from build123d import *

# Parameters (mm, degrees)
SKETCH1_W           = 12.1
SKETCH1_H           = 11.4
BOSS_EXTRUDE1_DEPTH = 500
SKETCH2_R           = 3.379
SKETCH2_R_2         = 1.9
CUT_EXTRUDE1_DEPTH  = 501.069087727
FILLET1_R           = 0.2


with BuildPart() as part:
    # Sketch1 → Boss-Extrude1 (new body)
    with BuildSketch(Plane.XY):
        Rectangle(SKETCH1_W, SKETCH1_H)
    extrude(amount=BOSS_EXTRUDE1_DEPTH)

    # Sketch2 → Cut-Extrude1 (cut, through all)
    with BuildSketch(Plane.XY.offset(500)):
        with Locations((0, 7.279)):
            Circle(SKETCH2_R)
        with Locations((0, -7.279)):
            Circle(SKETCH2_R)
        with Locations((-6.565, 2.930166572)):
            Circle(SKETCH2_R_2)
        with Locations((-6.565, -2.930166572)):
            Circle(SKETCH2_R_2)
        with Locations((6.565, -2.930166572)):
            Circle(SKETCH2_R_2)
        with Locations((6.565, 2.930166572)):
            Circle(SKETCH2_R_2)
    extrude(amount=-CUT_EXTRUDE1_DEPTH, mode=Mode.SUBTRACT)

    # Fillet1
    fillet1_edges = [part.edges().sort_by_distance(p)[0] for p in [
        (6.05, -4.759039176, 250),
        (6.05, -1.101293968, 250),
        (-6.05, -1.101293968, 250),
        (-6.05, -4.759039176, 250),
        (-6.05, 4.759039176, 250),
        (-6.05, 1.101293968, 250),
        (-2.987373428, -5.7, 250),
        (2.987373428, -5.7, 250),
        (6.05, 1.101293968, 250),
        (6.05, 4.759039176, 250),
        (2.987373428, 5.7, 250),
        (-2.987373428, 5.7, 250),
        (6.05, -5.7, 250),
        (-6.05, -5.7, 250),
        (-6.05, 5.7, 250),
        (6.05, 5.7, 250),
    ]]
    fillet(fillet1_edges, radius=FILLET1_R)


solid = part.part
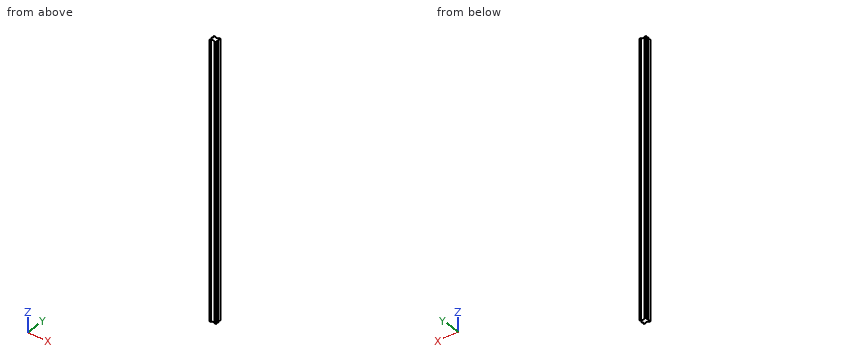
The listing builds one solid part. Answer for the finished solid, in the listing's coordinates (mm). Coordinates: 2 decimals unless noted, no trailing zeros. Write each loop counter-clockwise with the first axis right and the second up, starting at its lowest first coordinate (ties: lowest second). Pieces come first, ordered by that corner, then holes. Notation, with made-up numbers: M 82,76.5 L 140,76.5 A19 cw 140,87.5 Z; hole C 2.25,83.5 d7. An arc over 180 degrees is marked long. Put each result on its own line as item: value. Start each with the question number.
1. Consider line 1 (Y direction, x = 5.25, z = 328); line 2 (X direction, y = 2.75, z = 431); line 3 (Y direction, x = 5, z = 88). Determine where each line is inside the solid, lowest interval first. Write a range as from..to.
2. Flat-ended cylindrical pins translate along their axes: P1, Ø2, axis at x = 0.5, z = 193.5, coming from the -Y side; P2, Ø1, axis at x = 2, z = 192.5, coming from the +Y side. Find the tip coordinate at first contact, or state that the pin passes through.
3. A cutting plane is placed at B-B on x = 1. Write down the section's boundary in (y, z), then the cut area to 3 significant figures.
Resolved:
1. line 1: y = -5.7..-4.3, -1.56..1.56, 4.3..5.7
1. line 2: x = -4.67..4.67
1. line 3: y = -5.7..-4.01, -1.85..1.85, 4.01..5.7
2. P1: stops at y = -4.25
2. P2: stops at y = 5.01
3. outline: M -4.05,0 L 4.05,0 L 4.05,500 L -4.05,500 Z
3. area: 4,050 mm2
